Input: part model. Units: mm. Frame: model coordinates. A direction names the side the tool comes from. Give positions to 0.01 mm unless a question says otherwise; leave off trailing zeros. Loops run counter-clockwise (first coordinate to the right, second up) from the corner with the lowest first, then second, coordinate; pieces in that order, holes last. Notation, with made-up numbers: (33, 72) -> (77, 72) arc R17 ccw to (77, 90) -> close; hole circle Ø6 at (73.25, 6). An arc over 180 degrees is marked (long way). Answer as a JSON object with one key per item and string values.
```python
from build123d import *

# Parameters (mm, degrees)
EXTRUDE_2_DEPTH = 10
MM_1_D          = 3


with BuildPart() as part:
    # 草图3 → 凸台-拉伸2 (new body)
    with BuildSketch(Plane.XY):
        Polygon((-276.063392165, 169.449737011), (-276.063392165, -47.876740949), (-257.021298437, -66.918834677), (-125.22188191, -66.918834677), (-95.989685612, -47.876740949), (-95.989685612, 169.449737011), (-101.507171046, 174.967222445), (-115.03177934, 188.491830739), (-191.121590173, 169.449737011), (-257.328922186, 188.18420699), align=None)
    extrude(amount=EXTRUDE_2_DEPTH)

    # 大小mm 暗销孔1 (through all)
    with Locations(Plane(origin=(0, 0, 0), x_dir=(-1, 0, 0), z_dir=(0, 0, -1))):
        with Locations((170.910655251, 67.916631822), (228.522136285, 67.916631822), (228.522136285, -33.616473367), (170.910655251, -33.616473367)):
            Hole(MM_1_D / 2)


solid = part.part
```
Q1. Access query for faces 1 (the flat face through (-152.544, 179.104, 4.93)), 2 (the flat face through (-276.063, 62, 5)). Directions: +Z, -Z, +X, -X, +Y, -Y. A direction counts if a zero-diameter tool reaches every point of the face in a straight line with its end or side. Return the directions, or none.
Evaluation:
{"face 1": "+Z, -Z, +Y", "face 2": "+Z, -Z, -X, +Y, -Y"}
Q2. Section C-C, the plane x = -164.5. Return the cut outline in (y, z), then the cut area to 3 significant figures.
Evaluation:
{"outline": "(-66.92, 0) -> (176.11, 0) -> (176.11, 10) -> (-66.92, 10) -> close", "area": "2,430 mm2"}
Q3. Section B-B, the plane x = -109. Return the cut outline in (y, z), then the cut area to 3 significant figures.
Evaluation:
{"outline": "(-56.35, 0) -> (182.46, 0) -> (182.46, 10) -> (-56.35, 10) -> close", "area": "2,390 mm2"}
Q4. Pin query (flat end, axial travel): pin 1 (5 mm diameter, centred on x = -192, z = 7, fed in from +Y); pin 2 (2.5 mm diameter, centred on x = -170.91, y = -33.62, fed in from -Z). Return the tip coordinate at first contact, or that it passes through.
Evaluation:
{"pin 1": "stops at y = 170.41", "pin 2": "passes through"}
Q5. Section A-A, the plane z = 5. Return the cut outline in (x, y), then the cut area to 3 significant figures.
Evaluation:
{"outline": "(-276.06, -47.88) -> (-257.02, -66.92) -> (-125.22, -66.92) -> (-95.99, -47.88) -> (-95.99, 169.45) -> (-115.03, 188.49) -> (-191.12, 169.45) -> (-257.33, 188.18) -> (-276.06, 169.45) -> close; hole circle Ø3 at (-228.52, -33.62); hole circle Ø3 at (-228.52, 67.92); hole circle Ø3 at (-170.91, -33.62); hole circle Ø3 at (-170.91, 67.92)", "area": "43,800 mm2"}
Q6. Ray query, line 1 along Y through (x, z) = (-259, 3.5); line 2 along Y through (x, z) = (-165, 4.5). Return the intervals inside material, ascending.
Evaluation:
{"line 1": "y = -64.94 to 186.51", "line 2": "y = -66.92 to 175.99"}
